from build123d import *

# Parameters (mm, degrees)
SKETCH1_R           = 100
BOSS_EXTRUDE1_DEPTH = 10
BOSS_EXTRUDE1_TAPER = 40
SKETCH2_R           = 91.609003688
BOSS_EXTRUDE2_DEPTH = 10
BOSS_EXTRUDE2_TAPER = 60
FILLET1_R           = 10
FILLET2_R           = 2


# Read off the part's stored shape, not the designer's step: Shell1
with BuildPart() as part:
    # Sketch1 → Boss-Extrude1 (new body)
    with BuildSketch(Plane.XY):
        Circle(SKETCH1_R)
    extrude(amount=BOSS_EXTRUDE1_DEPTH, taper=BOSS_EXTRUDE1_TAPER)

    # Sketch2 → Boss-Extrude2 (add)
    with BuildSketch(Plane.XY.offset(10)):
        Circle(SKETCH2_R)
    extrude(amount=BOSS_EXTRUDE2_DEPTH, taper=BOSS_EXTRUDE2_TAPER)

    # Fillet1
    fillet1_edges = [part.edges().sort_by_distance(p)[0] for p in [
        (-91.609003688, 0, 10),
        (-74.288495613, 0, 20),
    ]]
    fillet(fillet1_edges, radius=FILLET1_R)

    # Fillet2
    fillet2_edges = [part.edges().sort_by_distance(p)[0] for p in [
        (-100, 0, 0),
    ]]
    fillet(fillet2_edges, radius=FILLET2_R)

    # Shell1 outline → Shell1 (revolve, cut)
    with BuildSketch(Plane.XZ):
        with BuildLine():
            Line((93.472963553, 0), (88.912189457, 5.435318914))
            ThreePointArc((88.912189457, 5.435318914), (88.29590529, 6.051603081), (87.581967242, 6.551507885))
            Line((87.581967242, 6.551507885), (74.109003688, 14.330127019))
            ThreePointArc((74.109003688, 14.330127019), (72.903098913, 14.829629131), (71.609003688, 15))
            Line((71.609003688, 15), (0, 15))
            Line((0, 15), (0, 0))
            Line((0, 0), (93.472963553, 0))
        make_face()
    revolve(axis=Axis((0, 0, 0), (0, 0, 1)), mode=Mode.SUBTRACT)


solid = part.part
Could you check a few things on this model? Use its own coordinates, in mm. Coordinates: 2 decimals unless noted, no trailing zeros.
Q1. Please list where these lines run through material, in increasing order: L1, parallel to Z at x = -38.5, y = 5.5; L2, parallel to X at y = -31.5, z = 5; L3, parallel to Y at x = 35.5, z = 14.
Q2. Thinking about a two-plate mould opening in X: for faces 1 (the flat face through (-1, 1, 20)), 2 (the flat face through (-1, 1, 15)), 3 (the conical face through (-61.313, -47.013, 18.283)), which applies, released by +X, released by -X, zero draft, split by the parting line, or undercut?
Q3. Will these pins go through, and if not, where does the flat tip stop? pin 1 (12 mm diameter, centred on y = -13, z = 6.5, fed in from +X); pin 2 (1.5 mm diameter, centred on x = -68, y = 31.5, fed in from +Z); pin 3 (12 mm diameter, centred on x = 75.5, z = 12.5, fed in from -Y).
Answer:
1. L1: z = 15 to 20
1. L2: x = -90.48 to -83.54, 83.54 to 90.48
1. L3: y = -76.88 to -65.7, 65.7 to 76.88
2. face 1: zero draft
2. face 2: undercut
2. face 3: split by the parting line
3. pin 1: stops at x = 97.3
3. pin 2: stops at z = 19.66
3. pin 3: stops at y = -59.88
